from build123d import *

# Parameters (mm, degrees)
F1_DEPTH = 812.8
F2_R     = 406.39999
F3_R     = 203.2
F4_DEPTH = 1016.001
F6_DEPTH = 812.8


# Not quite as in the source:
# - a fillet or chamfer is up to 0.001 mm smaller than in the source, because OpenCascade refuses the exact size


with BuildPart() as f1:
    # F0 (on Top) → F1 (new body)
    with BuildSketch(Plane.XY):
        Polygon((-69.4132745266, 217.2510341048), (-69.4132745266, -62.1489658952), (1251.3867254734, -62.1489658952), (1251.3867254734, 953.8510341048), (-69.4132745266, 953.8510341048), (-69.4132745266, 674.4510341048), (971.9867254734, 674.4510341048), (971.9867254734, 217.2510341048), align=None)
    extrude(amount=F1_DEPTH)

    # F2 (radius 406.4 in the source; OpenCascade refuses exactly that, so slightly less here)
    f2_edges = [f1.edges().sort_by_distance(p)[0] for p in [
        (-69.413275, 77.551034, 812.8),
        (-69.413275, 77.551034, 0),
        (-69.413275, 814.151034, 812.8),
        (-69.413275, 814.151034, 0),
    ]]
    fillet(f2_edges, radius=F2_R)

    # F3 (on face) → F4 (cut, through all)
    with BuildSketch(Plane.XZ.offset(62.1489658952)):
        with Locations((336.9867254734, 406.4)):
            Circle(F3_R)
    extrude(amount=-F4_DEPTH, mode=Mode.SUBTRACT)

    # F5 (on face) → F6 (join)
    with BuildSketch(Plane.YZ.offset(1251.3867254734)):
        with BuildLine():
            Line((445.8510341048, 177.8), (445.8510341048, 635))
            ThreePointArc((445.8510341048, 635), (217.2510341048, 406.4), (445.8510341048, 177.8))
        make_face()
        with BuildLine():
            ThreePointArc((674.4510341048, 406.4), (607.4956442841, 568.0446101792), (445.8510341048, 635))
            Line((445.8510341048, 635), (445.8510341048, 177.8))
            ThreePointArc((445.8510341048, 177.8), (607.4956442841, 244.7553898208), (674.4510341048, 406.4))
        make_face()
    extrude(amount=F6_DEPTH)


solid = f1.part
The listing builds one solid part. Answer for the finished solid, in the listing's coordinates (mm). A direction names the side the tool comes from. Coordinates: 2 decimals unless noted, no trailing zeros. Order: outer loops, then holes, each group sorted by start corner. A loop starts at its lowest first (then second) coordinate and runs counter-clockwise, first axis right, second up. Notation, with made-up numbers: (10, 49.5) -> (40, 49.5) arc R5 ccw to (40, 56.5) -> close; hole circle Ø3 at (67.25, 51.5). An arc over 180 degrees is marked (long way). Answer in a Markdown table with one row per item. Add a question column.
Item 1: Determine the mould class of faces 4 (the face through (46.476, 75.595, 122.209)), 5 (the face through (187.22, 812.2, 543.73)), 6 (the face through (2064.187, 443, 410)) for opening direction Z: +Z half, -Z half, draft (parallel to the pull), parting line (faces both ways), or undercut.
Item 2: Which of the six approach directions +Z, -Z, +X, -X, +Y, -Y give full straight-line access (tool end or side, diameter ignored) to faces 1 (the face through (46.476, 812.195, 690.591)), 2 (the face through (1251.387, 213, 401)), 3 (the face through (971.987, 449, 401))?
Item 3: Find section C-C (z = 93). Write down the section's boundary in (x, y).
Item 4: Find the intervals of material crossed by L1, parallel to X at y = 830, z = 406; L2, parallel to Y at x = 635, z = 756; L3, parallel to X at y = 455, z = 722, in increasing order. Write a range as from..to.
Item 5: Find section B-B (y = 295). Write down the section's boundary in (x, z), then the cut area to 3 significant figures.
Item 6: Find section A-A (z = 456). Write down the section's boundary in (x, y).
Item 7: Each of these flat-tipped pins is pushed along its axis until it touches: P1, Ø3, axis at y = 303, z = 437, coming from the -X side; P2, Ø1.5, axis at x = 1490.5, y = 479, coming from the +Z side; P3, Ø8, axis at y = 734, z = 603.5, coming from the -X side. Where does it stop, or does it pass through?
Item 8: Find section D-D (x = 1563.5). Write down the section's boundary in (y, z).
Result set:
| question | item | result |
|---|---|---|
| 1 | face 4 | -Z half |
| 1 | face 5 | undercut |
| 1 | face 6 | draft |
| 2 | face 1 | +Z, -X, +Y, -Y |
| 2 | face 2 | +X |
| 2 | face 3 | +Z, -Z, -X |
| 3 | outline | (78.26, -62.15) -> (1251.39, -62.15) -> (1251.39, 953.85) -> (78.26, 953.85) -> (78.26, 674.45) -> (971.99, 674.45) -> (971.99, 217.25) -> (78.26, 217.25) -> close |
| 4 | L1 | x = -69.41..133.79, 540.19..1251.39 |
| 4 | L2 | y = -62.15..217.25, 674.45..953.85 |
| 4 | L3 | x = 971.99..1251.39 |
| 5 | outline | (971.99, 0) -> (1251.39, 0) -> (1251.39, 234.64) -> (2064.19, 234.64) -> (2064.19, 578.16) -> (1251.39, 578.16) -> (1251.39, 812.8) -> (971.99, 812.8) -> close |
| 5 | area | 506,000 mm² |
| 6 | outline | (-66.38, -62.15) -> (139.93, -62.15) -> (139.93, 217.25) -> (-66.38, 217.25) -> close; (-66.38, 674.45) -> (139.93, 674.45) -> (139.93, 953.85) -> (-66.38, 953.85) -> close; (534.04, -62.15) -> (1251.39, -62.15) -> (1251.39, 222.7) -> (2064.19, 222.7) -> (2064.19, 669.01) -> (1251.39, 669.01) -> (1251.39, 953.85) -> (534.04, 953.85) -> (534.04, 674.45) -> (971.99, 674.45) -> (971.99, 217.25) -> (534.04, 217.25) -> close |
| 7 | P1 | stops at x = 971.99 |
| 7 | P2 | stops at z = 632.69 |
| 7 | P3 | stops at x = -20.61 |
| 8 | outline | circle Ø457.2 at (445.85, 406.4) |
